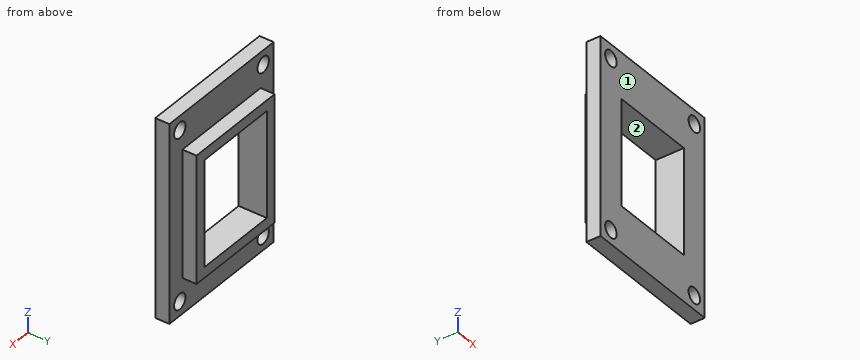
```python
from build123d import *

# Parameters (mm, degrees)
SKETCH1_W           = 19.05
SKETCH1_H           = 22.86
SKETCH1_W_2         = 15.24
SKETCH1_H_2         = 19.05
BOSS_EXTRUDE1_DEPTH = 5.08
SKETCH3_W           = 25.4
SKETCH3_H           = 35.56
SKETCH3_R           = 1.397
SKETCH3_W_2         = 19.05
SKETCH3_H_2         = 22.86
BOSS_EXTRUDE2_DEPTH = 2.54


with BuildPart() as part:
    # Sketch1 → Boss-Extrude1 (new body)
    with BuildSketch(Plane(origin=(0, 0, 0), x_dir=(1, 0, 0), z_dir=(0, 1, 0))):
        Rectangle(SKETCH1_W, SKETCH1_H)
        Rectangle(SKETCH1_W_2, SKETCH1_H_2, mode=Mode.SUBTRACT)
    extrude(amount=BOSS_EXTRUDE1_DEPTH)

    # Sketch3 → Boss-Extrude2 (add)
    with BuildSketch(Plane(origin=(0, 0, 0), x_dir=(1, 0, 0), z_dir=(0, 1, 0))):
        Rectangle(SKETCH3_W, SKETCH3_H)
        with Locations(Location((-10.16, 15.24, 0), (0, 0, 270))):
            Circle(SKETCH3_R, mode=Mode.SUBTRACT)
        with Locations(Location((10.16, 15.24, 0), (0, 0, 90))):
            Circle(SKETCH3_R, mode=Mode.SUBTRACT)
        with Locations(Location((-10.16, -15.24, 0), (0, 0, 90))):
            Circle(SKETCH3_R, mode=Mode.SUBTRACT)
        with Locations(Location((10.16, -15.24, 0), (0, 0, 270))):
            Circle(SKETCH3_R, mode=Mode.SUBTRACT)
        Rectangle(SKETCH3_W_2, SKETCH3_H_2, mode=Mode.SUBTRACT)
    extrude(amount=BOSS_EXTRUDE2_DEPTH)


solid = part.part
```
Here's how the part is built. I have some questions about the finished solid (model axes, mm). Face numbers are marked on the shaded views. Coordinates: 2 decimals unless noted, no trailing zeros. Order: outer loops, then holes, each group sorted by start corner. A loop starts at its lowest first (then second) coordinate and runs counter-clockwise, first axis right, second up. Notation, with made-up numbers: (54, 48.25) - (60, 48.25) arc R26 cw to (60, 64.25) - close; hole circle Ø5 at (43, 30.25). An arc over 180 degrees is marked (long way). One line per question, with ' | ' between items. Start each with the question number.
1. If we section it at A-A (z = -15.24): Write out the boundary of the cut face in (x, y), and give its area (3 significant figures).
2. If we section it at C-C (y = 1.6): Write out the boundary of the cut face in (x, z) (3 decimals), and give its area (3 significant figures).
3. If we mould it in two halves opening along Z, with no side actions, what happens to the marked faces 1 and 2? For each: released by +Z, released by -Z, zero draft, split by the parting line, or undercut.
4. I'm going to push flat-ended pins straight in: pin 1 Ø4.5 at (x, z) = (10.16, 15.24) entering from +Y; pin 2 Ø0.8 at (x, y) = (0, 4) entering from +Z; pin 3 Ø0.8 at (x, y) = (-4.5, 3.5) entering from -Z. Where does each tip first touch, or does it pass through?
5. If we section it at B-B (x = 10.16): Write out the boundary of the cut face in (y, z).
6. If we section it at D-D (y = 3.3): Write out the boundary of the cut face in (x, z) (3 decimals).
7. Please list where these lines run through material, in increasing order: line 1 along Z through (x, y) = (2.25, 0.95) (3 decimals); line 2 along X through (y, z) = (3.6, -4) (3 decimals); line 3 along Z through (x, y) = (-5, 4) (3 decimals). Write a range as [from, to].
Model answer:
1) outline: (-12.7, 0) - (-11.56, 0) - (-11.56, 2.54) - (-12.7, 2.54) - close; (-8.76, 0) - (8.76, 0) - (8.76, 2.54) - (-8.76, 2.54) - close; (11.56, 0) - (12.7, 0) - (12.7, 2.54) - (11.56, 2.54) - close | area: 50.3 mm²
2) outline: (-12.7, -17.78) - (12.7, -17.78) - (12.7, 17.78) - (-12.7, 17.78) - close; hole circle Ø2.794 at (-10.16, -15.24); hole circle Ø2.794 at (-10.16, 15.24); hole (-7.62, -9.525) - (7.62, -9.525) - (7.62, 9.525) - (-7.62, 9.525) - close; hole circle Ø2.794 at (10.16, -15.24); hole circle Ø2.794 at (10.16, 15.24) | area: 588 mm²
3) face 1: zero draft | face 2: undercut
4) pin 1: stops at y = 2.54 | pin 2: stops at z = 11.43 | pin 3: stops at z = -11.43
5) outline: (0, -17.78) - (2.54, -17.78) - (2.54, -16.64) - (0, -16.64) - close; (0, -13.84) - (2.54, -13.84) - (2.54, 13.84) - (0, 13.84) - close; (0, 16.64) - (2.54, 16.64) - (2.54, 17.78) - (0, 17.78) - close
6) outline: (-9.525, -11.43) - (9.525, -11.43) - (9.525, 11.43) - (-9.525, 11.43) - close; hole (-7.62, -9.525) - (7.62, -9.525) - (7.62, 9.525) - (-7.62, 9.525) - close
7) line 1: z = [-17.78, -9.525], [9.525, 17.78] | line 2: x = [-9.525, -7.62], [7.62, 9.525] | line 3: z = [-11.43, -9.525], [9.525, 11.43]
